Here's how the part is built. I have some questions about the finished solid (model axes, mm). Coordinates: 2 decimals unless noted, no trailing zeros. Write each loop counter-clockwise with the first axis right and the second up, starting at its lowest first coordinate (ties: lowest second). Pieces come first, ordered by that corner, then holes. Notation, with made-up numbers: M 49,11 L 62,11 A18 cw 62,24 Z; hole C 78,42 d6. An arc over 180 degrees is marked long. Use a Markdown table: item, result.
```python
from build123d import *

# Parameters (mm, degrees)
EXTRUDE_1_DEPTH     = 6
SKETCH_2_R          = 1.25
CUT_EXTRUDE_1_DEPTH = 10
SKETCH_3_R          = 1.05
CUT_EXTRUDE_2_DEPTH = 81.845531726
SKETCH_4_R          = 2.55
CUT_EXTRUDE_3_DEPTH = 81.845531783
SKETCH_5_W          = 8
SKETCH_5_H          = 6
EXTRUDE_2_DEPTH     = 20
FILLET_2_R          = 10
FILLET_3_R          = 10
SKETCH_7_R          = 1.55
EXTRUDE_3_DEPTH     = 6
FILLET_4_R          = 8
SKETCH_9_W          = 9
SKETCH_9_H          = 6
EXTRUDE_4_DEPTH     = 3.5


with BuildPart() as part:
    # ｽｹｯﾁ1 → ﾎﾞｽ - 押し出し1 (new body)
    with BuildSketch(Plane(origin=(0, 0, 0), x_dir=(1, 0, 0), z_dir=(0, 1, 0))):
        Polygon((0, -70), (0, 70), (36.5, 70), (36.5, 61), (40, 61), (40, 45), (20, 45), (20, -45), (40, -45), (40, -61), (36.5, -61), (36.5, -70), align=None)
    extrude(amount=EXTRUDE_1_DEPTH)

    # ｽｹｯﾁ2 → ｶｯﾄ - 押し出し1 (cut)
    with BuildSketch(Plane(origin=(40, 0, 0), x_dir=(0, 0, -1), z_dir=(1, 0, 0))):
        with Locations((48, 3)):
            Circle(SKETCH_2_R)
        with Locations((58, 3)):
            Circle(SKETCH_2_R)
        with Locations(Location((-48, 3, 0), (0, 0, 180))):
            Circle(SKETCH_2_R)
        with Locations(Location((-58, 3, 0), (0, 0, 180))):
            Circle(SKETCH_2_R)
    extrude(amount=-CUT_EXTRUDE_1_DEPTH, mode=Mode.SUBTRACT)

    # ｽｹｯﾁ3 → ｶｯﾄ - 押し出し2 (cut, through all)
    with BuildSketch(Plane(origin=(0, 6, 0), x_dir=(1, 0, 0), z_dir=(0, 1, 0))):
        with Locations((40.7, 58)):
            Circle(SKETCH_3_R)
        with Locations((40.7, 48)):
            Circle(SKETCH_3_R)
        with Locations((40.7, -48)):
            Circle(SKETCH_3_R)
        with Locations((40.7, -58)):
            Circle(SKETCH_3_R)
    extrude(amount=-CUT_EXTRUDE_2_DEPTH, mode=Mode.SUBTRACT)

    # ｽｹｯﾁ4 → ｶｯﾄ - 押し出し3 (cut, through all)
    with BuildSketch(Plane(origin=(0, 6, 0), x_dir=(1, 0, 0), z_dir=(0, 1, 0))):
        with Locations(Location((10, 0, 0), (0, 0, 270))):
            Circle(SKETCH_4_R)
        with Locations(Location((10, 60, 0), (0, 0, 270))):
            Circle(SKETCH_4_R)
        with Locations(Location((10, -60, 0), (0, 0, 270))):
            Circle(SKETCH_4_R)
    extrude(amount=-CUT_EXTRUDE_3_DEPTH, mode=Mode.SUBTRACT)

    # ｽｹｯﾁ5 → ﾎﾞｽ - 押し出し2 (add)
    with BuildSketch(Plane(origin=(20, 0, 0), x_dir=(0, 0, -1), z_dir=(1, 0, 0))):
        with Locations((0, 3)):
            Rectangle(SKETCH_5_W, SKETCH_5_H)
    extrude(amount=EXTRUDE_2_DEPTH)

    # ﾌｨﾚｯﾄ2
    fillet_2_edges = [part.edges().sort_by_distance(p)[0] for p in [
        (20, 3, 4),
        (20, 3, -4),
    ]]
    fillet(fillet_2_edges, radius=FILLET_2_R)

    # ﾌｨﾚｯﾄ3
    fillet_3_edges = [part.edges().sort_by_distance(p)[0] for p in [
        (0, 3, 70),
        (0, 3, -70),
    ]]
    fillet(fillet_3_edges, radius=FILLET_3_R)

    # ｽｹｯﾁ7 → ﾎﾞｽ - 押し出し3 (add, through all)
    # profile 1 of 2: a face of its own
    with BuildSketch(Plane(origin=(0, 6, 0), x_dir=(1, 0, 0), z_dir=(0, 1, 0))):
        with BuildLine():
            Line((23.5, 28.25), (20, 28.25))
            Line((20, 28.25), (20, 21.75))
            Line((20, 21.75), (23.5, 21.75))
            ThreePointArc((23.5, 21.75), (26.75, 25), (23.5, 28.25))
        make_face()
        with Locations(Location((23.5, 25, 0), (0, 0, 270))):
            Circle(SKETCH_7_R, mode=Mode.SUBTRACT)
    # profile 2 of 2: a face of its own
    with BuildSketch(Plane(origin=(0, 6, 0), x_dir=(1, 0, 0), z_dir=(0, 1, 0))):
        with BuildLine():
            Line((20, -21.75), (23.5, -21.75))
            ThreePointArc((23.5, -21.75), (26.75, -25), (23.5, -28.25))
            Line((23.5, -28.25), (20, -28.25))
            Line((20, -28.25), (20, -21.75))
        make_face()
        with Locations(Location((23.5, -25, 0), (0, 0, 90))):
            Circle(SKETCH_7_R, mode=Mode.SUBTRACT)
    extrude(amount=-EXTRUDE_3_DEPTH)

    # ﾌｨﾚｯﾄ4
    fillet_4_edges = [part.edges().sort_by_distance(p)[0] for p in [
        (20, 3, 28.25),
        (20, 3, 21.75),
        (20, 3, -28.25),
        (20, 3, -21.75),
    ]]
    fillet(fillet_4_edges, radius=FILLET_4_R)

    # ｽｹｯﾁ9 → ﾎﾞｽ - 押し出し4 (add)
    with BuildSketch(Plane(origin=(36.5, 0, 0), x_dir=(0, 0, -1), z_dir=(1, 0, 0))):
        with Locations((-65.5, 3)):
            Rectangle(SKETCH_9_W, SKETCH_9_H)
        with Locations((65.5, 3)):
            Rectangle(SKETCH_9_W, SKETCH_9_H)
    extrude(amount=EXTRUDE_4_DEPTH)


solid = part.part
```
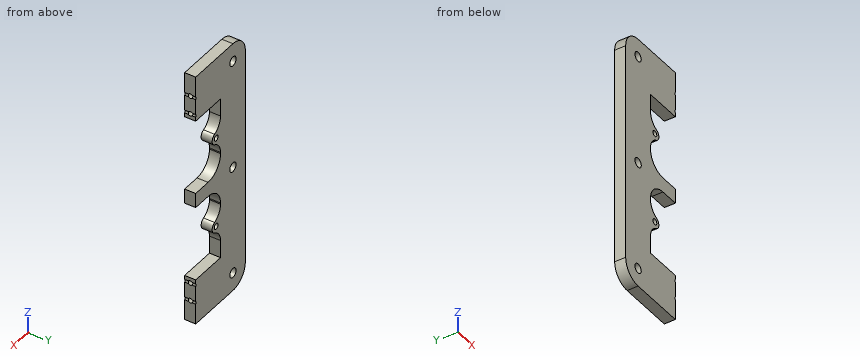
1. I need wall thicknesses on probe 1 along Z at (x, y) = (37, 1); probe 2 along Z at (x, y) = (9, 5.25); probe 3 along Y at (x, z) = (33, 48). Which ranges of each line are inside material? Lowest first, please.
Answers follow:
| item | result |
|---|---|
| probe 1 | z = -70 to -45, -4 to 4, 45 to 70 |
| probe 2 | z = -69.95 to -62.35, -57.65 to -2.35, 2.35 to 57.65, 62.35 to 69.95 |
| probe 3 | y = 0 to 1.75, 4.25 to 6 |
2. Suppose I cut it at C-C on y = 3. State how many separate pieces and enclosed holes the cut face has, and give its area (3 significant figures).
Answers follow:
| item | result |
|---|---|
| separate pieces | 1 |
| enclosed holes | 5 |
| area | 3,900 mm2 |
3. Will this pin go through, and if not, where does the flat tip stop? pin 1 Ø0.6 at (y, z) = (3.5, 14) entering from +X.
Answers follow:
| item | result |
|---|---|
| pin 1 | stops at x = 20 |
4. Suppose I cut it at A-A on x = 32. Write out the boundary of the cut face in (y, z).
Answers follow:
| item | result |
|---|---|
| outline | M 0,-70 L 6,-70 L 6,-45 L 0,-45 Z; M 0,-4 L 6,-4 L 6,4 L 0,4 Z; M 0,45 L 6,45 L 6,70 L 0,70 Z; hole C 3,-58 d2.5; hole C 3,-48 d2.5; hole C 3,48 d2.5; hole C 3,58 d2.5 |
5. Suppose I cut it at B-B on z = 25. Write out the boundary of the cut face in (x, y).
Answers follow:
| item | result |
|---|---|
| outline | M 0,0 L 21.95,0 L 21.95,6 L 0,6 Z; M 25.05,0 L 26.75,0 L 26.75,6 L 25.05,6 Z |
6. Suppose I cut it at D-D on z = 40.5. Write out the boundary of the cut face in (x, y), and give its area (3 significant figures).
Answers follow:
| item | result |
|---|---|
| outline | M 0,0 L 20,0 L 20,6 L 0,6 Z |
| area | 120 mm2 |
